Part model, mm, in its own coordinate system. A direction names the side the tool comes from. Round coordinates to 2 decimals unless told otherwise and drop trailing zeros. Loops run counter-clockwise (first coordinate to the right, second up) from the corner with the lowest first, then second, coordinate; pieces in that order, holes last.
1) 3-axis set-ups, long thin cutter, end or side, ignore diameter. For faces 5 (the flat face through (-33, -3, 0)), 6 (the flat face through (-8, 39.204, 5)), 7 (the cylindrical face through (-32.492, 0.715, -4.93)): which of +Z, -Z, +X, -X, +Y, -Y reach the whole face in a straight line?
2) Mould opens along X. For faces 1 (the cylindrical face through (-8.401, 54.716, -5.07)), 2 (the flat face through (0, -39, -2)), 3 (the flat face through (-16.411, 49, -5)), 4 (the flat face through (-8, 49, 0)) say: +X half, -X half, draft (parallel to the pull), parting line (faces both ways), or undercut.
3) Band-saw the part on D-D, the plane y = 27.5. Write the cut outline in (x, z).
4) Band-saw the part on A-A, the plane x = -24.5. Write the cut outline in (y, z), then the cut area to 3 significant figures.
5) Drop flat-ended pins along their axis: P1, Ø5, axis at y = 47.5, z = -2.5, coming from the -X side; P2, Ø5, axis at x = -10, y = 49.5, coming from the +Z side; P3, Ø10, axis at y = -25.5, z = 3, coming from the -X side. Give the stop position or say it passes through.
6) Band-saw the part on B-B, the plane y = 0. Write the cut outline in (x, z), then the cut area to 3 significant figures.
7) Band-saw the part on C-C, the plane z = 2.5. Write the cut outline in (x, y), then the cut area to 3 significant figures.
8) Probe line 1 (Y direction, x = -16, z = -4.75); line 2 (Y direction, x = -3.5, z = 0.75); line 3 (X direction, y = 45.5, z = -7). List the from-to ranges inside material, lowest first.
Autodesk Inventor part; units mm, degrees
ref_plane "YZ Plane" through (0, 0, 0) normal (1, 0, 0) x (0, 1, 0)
ref_plane "XZ Plane" through (0, 0, 0) normal (0, 1, 0) x (-1, 0, 0)
ref_plane "XY Plane" through (0, 0, 0) normal (0, 0, 1) x (1, 0, 0)
sketch "草圖1" plane through (0, 0, 0) normal (0, 0, 1) x (1, 0, 0)
  arc A0 (0, 32.5) -> (0, -32.5) centre (0, 0) ccw
  arc A1 (0, 37.5) -> (0, -37.5) centre (0, 0) ccw
  arc A2 (0, 42.5) -> (0, -42.5) centre (0, 0) ccw
  line L0 (0, 0) -> (0, -59.8463)
  line L1 (0, -59.8463) -> (0, 72.1748)
  point P0 (0, -37.5)
  point P1 (0, -42.5)
  dimension "d22" = 32.5
  dimension "d23" = 37.5
  dimension "d24" = 42.5
extrude "擠出1" add sketch "草圖1" against normal blind 10 contours A0 L0 A1 L1
extrude "擠出2" add sketch "草圖1" along normal mid plane 20 contours A1 L0 A2 L1
sketch "草圖2" plane through (0, 0, -10) normal (0, 0, -1) x (1, 0, 0)
  line L0 (0, -42.5) -> (0, -32.5)
  line L1 (0, -42.5) -> (0, -32.5)
  arc A0 (0, 42.5) -> (0, -42.5) centre (0, 0) ccw
  line L2 (-16.4109, -59.2037) -> (0, -59.2037)
  line L3 (0, -59.2037) -> (0, -42.5)
  line L4 (-16.4109, -39.2037) -> (-16.4109, -59.2037)
  dimension "d4" = 10
  dimension "d16" = 20
extrude "擠出3" add sketch "草圖2" against normal blind 20
sketch "草圖4" plane through (0, 0, -10) normal (0, 0, -1) x (1, 0, 0)
  line L0 (3, 24.6083) -> (3, 21.6083)
  line L1 (0, -59.2037) -> (0, -32.5)
  line L2 (0, 21.6083) -> (3, 21.6083)
  circle A0 centre (3, 21.6083) radius 1.5
  line L3 (0, -59.2037) -> (-16.4109, -59.2037)
  line L4 (-16.4109, -59.2037) -> (-8.2055, -59.2037)
  line L5 (-8.2055, -56.2037) -> (-8.2055, -59.2037)
  line L6 (-16.4109, -59.2037) -> (-16.4109, -39.2037)
  circle A1 centre (-8.2055, -56.2037) radius 1.5
  point P0 (0, 0)
  point P1 (0, 24.3333)
  point P2 (0, 13.1972)
  point P3 (0, -15.5384)
  dimension "d10" = 3
  dimension "d11" = 3
  dimension "d12" = 3
  dimension "d17" = 3
  dimension "d18" = 3
extrude "擠出4" cut sketch "草圖4" against normal blind 20 contours A1
sketch "草圖6" plane through (-16.4109, 39.2037, -10) normal (-1, 0, 0) x (0, 0, 1)
  line L0 (0, 20) -> (20, 20)
  line L1 (20, 20) -> (10, 20)
  line L2 (10, 20) -> (10, 0)
  line L3 (20, 0) -> (0, 0)
  line L4 (20, 20) -> (20, 0)
  line L5 (10, 20) -> (20, 20)
  line L6 (20, 20) -> (20, 0)
  line L7 (20, 0) -> (10, 0)
  line L8 (10, 0) -> (10, 20)
  point P0 (10, -39.2037)
  dimension "d19" = 10
extrude "擠出5" cut sketch "草圖6" against normal blind 20
properties part number "ARML"
Reported:
1. face 5: +Z, +X
1. face 6: +Z, +X, -X, +Y
1. face 7: +Z, -Z, +X
2. face 1: undercut
2. face 2: +X half
2. face 3: -X half
2. face 4: draft
3. outline: (-32.4, -10) - (-17.32, -10) - (-17.32, 0) - (-25.5, 0) - (-25.5, 10) - (-32.4, 10) - close
4. outline: (-34.73, -10) - (-21.35, -10) - (-21.35, 0) - (-28.39, 0) - (-28.39, 10) - (-34.73, 10) - close; (21.35, -10) - (34.73, -10) - (34.73, 10) - (28.39, 10) - (28.39, 0) - (21.35, 0) - close
4. area: 394 mm2
5. P1: stops at x = -16.41
5. P2: stops at z = 0
5. P3: stops at x = -37.23
6. outline: (-42.5, -10) - (-32.5, -10) - (-32.5, 0) - (-37.5, 0) - (-37.5, 10) - (-42.5, 10) - close
6. area: 150 mm2
7. outline: (-16.41, 39.2) arc R42.5 ccw to (0, -42.5) - (0, -37.5) arc R37.5 cw to (0, 37.5) - (0, 39.2) - close
7. area: 592 mm2
8. line 1: y = -39.37 to -28.29, 28.29 to 59.2
8. line 2: y = -42.36 to -37.34, 37.34 to 39.2
8. line 3: x = -16.41 to 0
